```python
from build123d import *

# Parameters (mm, degrees)
SKETCH_1_W          = 50
SKETCH_1_H          = 15
EXTRUDE_1_DEPTH     = 5
SKETCH_2_W          = 40
SKETCH_2_H          = 5
EXTRUDE_3_DEPTH     = 12
SKETCH_3_R          = 9
SKETCH_3_R_2        = 1.5
CUT_EXTRUDE_1_DEPTH = 16


with BuildPart() as part:
    # 草图1 → 凸台-拉伸1 (new body)
    with BuildSketch(Plane.ZY):
        Rectangle(SKETCH_1_W, SKETCH_1_H)
        with BuildLine():
            Line((-16, 2.5), (16, 2.5))
            ThreePointArc((16, 2.5), (18.5, 0), (16, -2.5))
            Line((16, -2.5), (-16, -2.5))
            ThreePointArc((-16, -2.5), (-18.5, 0), (-16, 2.5))
        make_face(mode=Mode.SUBTRACT)
    extrude(amount=EXTRUDE_1_DEPTH)

    # 草图2 → 凸台-拉伸3 (add)
    with BuildSketch(Plane(origin=(0, 0, 0), x_dir=(0, 0, -1), z_dir=(1, 0, 0))):
        with Locations((0, 5)):
            Rectangle(SKETCH_2_W, SKETCH_2_H)
    extrude(amount=EXTRUDE_3_DEPTH)

    # 草图3 → 切除-拉伸1 (cut, through all)
    with BuildSketch(Plane(origin=(0, 7.5, 0), x_dir=(1, 0, 0), z_dir=(0, 1, 0))):
        with Locations((15, 0)):
            Circle(SKETCH_3_R)
        with Locations((6, 14)):
            Circle(SKETCH_3_R_2)
        with Locations((6, -14)):
            Circle(SKETCH_3_R_2)
    extrude(amount=-CUT_EXTRUDE_1_DEPTH, mode=Mode.SUBTRACT)


solid = part.part
```
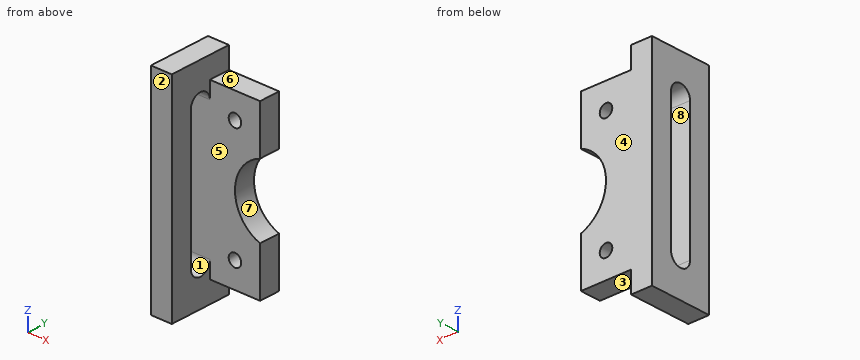
Input: part model. Units: mm. Frame: model coordinates. Face numbers are marked on the shaded views. A direction names the side the tool comes from. Coordinates: 2 decimals unless noted, no trailing zeros. Loops run counter-clockwise (first coordinate to the right, second up) from the corner with the lowest first, then second, coordinate; pieces in that order, holes last. Notation, with made-up numbers: M 50.5,47.5 L 75.5,47.5 A5 ccw 75.5,54.5 Z; hole C 80.5,82 d8. An arc over 180 degrees is marked long. One line per item, written item: value.
(1) Pull-direction query (Y, two-part tool) for the marked faces 1, 2, 3 and 4; classes: +Y half, -Y half, draft (parallel to the pull), parting line (faces both ways), or undercut.
Filled in:
face 1: undercut
face 2: -Y half
face 3: draft
face 4: +Y half
(2) Section A-A (y = 0). Output: boundary loops of the cut face in (x, z).
Filled in:
outline: M -5,-25 L 0,-25 L 0,-18.5 L -5,-18.5 Z; M -5,18.5 L 0,18.5 L 0,25 L -5,25 Z
(3) Reachability of the marked faces 5, 6, 7 and 8 from +Z, -Z, +X, -X, +Y, -Y: full face, straight path, thin tool, end or side. Return the list, or none.
Filled in:
face 5: +X
face 6: +Z, +X, +Y, -Y
face 7: +X, +Y, -Y
face 8: +X, -X
(4) Section D-D (z = -9). Output: boundary loops of the cut face in (x, y).
Filled in:
outline: M -5,-7.5 L 0,-7.5 L 0,-2.5 L -5,-2.5 Z; M -5,2.5 L 12,2.5 L 12,7.5 L -5,7.5 Z
(5) Section C-C (y = 6.5). Output: boundary loops of the cut face in (x, z).
Filled in:
outline: M -5,-25 L 0,-25 L 0,-20 L 12,-20 L 12,-8.49 A9 cw 12,8.49 L 12,20 L 0,20 L 0,25 L -5,25 Z; hole C 6,-14 d3; hole C 6,14 d3
(6) Section B-B (z = 14). Output: boundary loops of the cut face in (x, y), and give its area (3 significant figures).
Filled in:
outline: M -5,-7.5 L 0,-7.5 L 0,-2.5 L -5,-2.5 Z; M -5,2.5 L 4.5,2.5 L 4.5,7.5 L -5,7.5 Z; M 7.5,2.5 L 12,2.5 L 12,7.5 L 7.5,7.5 Z
area: 95.0 mm^2
(7) Line query: line 1 along Y through (x, z) = (-1.5, -13); line 2 along X through (y, z) = (4.5, -14); line 3 along Y through (x, z) = (6, 4.5). Output: solid intervals per line, ascending. Write a range as from..to.
Filled in:
line 1: -7.5..-2.5, 2.5..7.5
line 2: -5..4.5, 7.5..12
line 3: 2.5..7.5
(8) Pin query (flat end, axial travel): pin 1 (1.5 mm diameter, centred on x = 2, z = 3.5, fed in from -Y); pin 2 (1 mm diameter, centred on y = -3, z = 18.5, fed in from +X); pin 3 (5.5 mm diameter, centred on x = 5.5, y = 6, fed in from -Z). Return the tip coordinate at first contact, or that it passes through.
Filled in:
pin 1: y = 2.5
pin 2: x = 0
pin 3: z = -20
